```python
from build123d import *

# Parameters (mm, degrees)
F3_DEPTH = 6.5


with BuildPart() as f1:
    # F0 (on Front) → F1 (revolve)
    with BuildSketch(Plane.XZ):
        Polygon((4, -2.5), (4, 0), (2.5, -6.5), (2.5, -15.5), (4, -20.5), (4, -15.5), (6, -15.5), (15.640222, -5.859778), align=None)
    revolve(axis=Axis((0, 0, 0.112359), (0, 0, -1)))

    # F2 (on Front) → F3 (intersect, symmetric)
    with BuildSketch(Plane.XZ):
        Polygon((6.5, 0), (4, 0), (-4, 0), (-6.5, 0), (-6.5, -10.5), (-4.75, -15.5), (-4.75, -20.5), (0, -20.5), (4.75, -20.5), (4.75, -15.5), (6.5, -10.5), align=None)
    extrude(amount=F3_DEPTH, both=True, mode=Mode.INTERSECT)


solid = f1.part
```
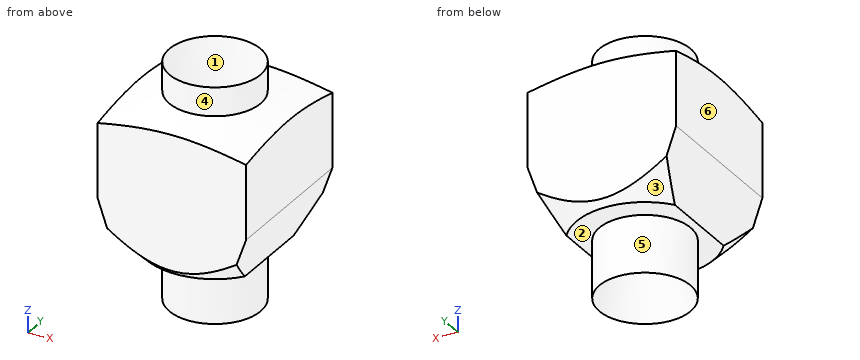
Geometry check sheet. Reference: the model listing, model coordinates, mm. Face numbers are marked on the shaded views. A direction names the side the tool comes from. Coordinates: 2 decimals unless noted, no trailing zeros. Order: outer loops, then holes, each group sorted by start corner. A loop starts at its lowest first (then second) coordinate and runs counter-clockwise, first axis right, second up.
Q1. Sectioned sample at A-A on x = 0. Record the cut outline in (y, z), and give its area (3 significant figures).
Reply:
outline: (-6.5, -15) - (-6, -15.5) - (-4, -15.5) - (-4, -20.5) - (-2.5, -15.5) - (-2.5, -6.5) - (-4, 0) - (-4, -2.5) - (-6.5, -3.22) - close; (2.5, -15.5) - (4, -20.5) - (4, -15.5) - (6, -15.5) - (6.5, -15) - (6.5, -3.22) - (4, -2.5) - (4, 0) - (2.5, -6.5) - close
area: 107 mm2
Q2. Depth check by flat-ended pin: pin 1 Ø3 at (x, y) = (-4, 4) entering from -Z; pin 2 Ø5 at (y, z) = (-4.5, -15.5) entering from -X (3 decimals). Enter the tip coordinate at first touch or a pass-through.
Reply:
pin 1: stops at z = -15.5
pin 2: stops at x = -5.625
Q3. Thickness scan on probe 1 along X at (y, z) = (0, -8.5); probe 2 along Y at (x, z) = (-2.25, -6). Record the ranges inside material, lowest first.
Reply:
probe 1: x = -6.5 to -2.5, 2.5 to 6.5
probe 2: y = -6.5 to -1.33, 1.33 to 6.5
Q4. Sectioned sample at C-C on z = -6.25. Record the cut outline in (x, y).
Reply:
outline: (-6.5, -6.5) - (6.5, -6.5) - (6.5, 6.5) - (-6.5, 6.5) - close; hole circle Ø5.12 at (0, 0)
Q5. Sectioned sample at B-B on y = 0. Record the cut outline in (x, z), and give its area (3 significant figures).
Reply:
outline: (-6.5, -10.5) - (-4.75, -15.5) - (-4, -15.5) - (-4, -20.5) - (-2.5, -15.5) - (-2.5, -6.5) - (-4, 0) - (-4, -2.5) - (-6.5, -3.22) - close; (2.5, -15.5) - (4, -20.5) - (4, -15.5) - (4.75, -15.5) - (6.5, -10.5) - (6.5, -3.22) - (4, -2.5) - (4, 0) - (2.5, -6.5) - close
area: 98.7 mm2
Q6. Tool access check on the marked faces 4, 5 and 6. Record the directions out of +Z, -Z, +X, -X, +Y, -Y that give a thin tool (end or side, any length) a straight path to the whole face; none if there is none.
Reply:
face 4: +Z
face 5: -Z
face 6: +Z, -Z, -X, +Y, -Y
Q7. Draft check along X on the marked faces 1, 2 and 3. Enter one of: released by +X, released by -X, zero draft, split by the parting line, or undercut.
Reply:
face 1: undercut
face 2: zero draft
face 3: split by the parting line
Q8. Sectioned sample at D-D on z = -13.5. Record the cut outline in (x, y).
Reply:
outline: (-5.45, -5.86) arc R8 ccw to (-4.66, -6.5) - (4.66, -6.5) arc R8 ccw to (5.45, -5.86) - (5.45, 5.86) arc R8 ccw to (4.66, 6.5) - (-4.66, 6.5) arc R8 ccw to (-5.45, 5.86) - close; hole circle Ø5 at (0, 0)
